Autodesk Fusion 360 part; units mm, degrees
sketch "Boceto1" plane through (0, 0, 0) normal (0, 1, 0) x (1, 0, 0)
  line L0 (3.025, -2.525) -> (16.025, -2.525)
  line L1 (3.025, -16.525) -> (16.025, -16.525)
  line L2 (2.525, -3.025) -> (2.525, -16.025)
  line L3 (16.525, -3.025) -> (16.525, -16.025)
  arc A0 (3.025, -2.525) -> (2.525, -3.025) centre (3.025, -3.025) ccw
  arc A1 (16.525, -3.025) -> (16.025, -2.525) centre (16.025, -3.025) ccw
  arc A2 (2.525, -16.025) -> (3.025, -16.525) centre (3.025, -16.025) ccw
  arc A3 (16.025, -16.525) -> (16.525, -16.025) centre (16.025, -16.025) ccw
  line L4 (22.075, -2.525) -> (35.075, -2.525)
  line L5 (22.075, -16.525) -> (35.075, -16.525)
  line L6 (21.575, -3.025) -> (21.575, -16.025)
  line L7 (35.575, -3.025) -> (35.575, -16.025)
  arc A4 (22.075, -2.525) -> (21.575, -3.025) centre (22.075, -3.025) ccw
  arc A5 (35.575, -3.025) -> (35.075, -2.525) centre (35.075, -3.025) ccw
  arc A6 (21.575, -16.025) -> (22.075, -16.525) centre (22.075, -16.025) ccw
  arc A7 (35.075, -16.525) -> (35.575, -16.025) centre (35.075, -16.025) ccw
  line L8 (3.025, -21.575) -> (16.025, -21.575)
  line L9 (3.025, -35.575) -> (16.025, -35.575)
  line L10 (2.525, -22.075) -> (2.525, -35.075)
  line L11 (16.525, -22.075) -> (16.525, -35.075)
  arc A8 (3.025, -21.575) -> (2.525, -22.075) centre (3.025, -22.075) ccw
  arc A9 (16.525, -22.075) -> (16.025, -21.575) centre (16.025, -22.075) ccw
  arc A10 (2.525, -35.075) -> (3.025, -35.575) centre (3.025, -35.075) ccw
  arc A11 (16.025, -35.575) -> (16.525, -35.075) centre (16.025, -35.075) ccw
  line L12 (22.075, -21.575) -> (35.075, -21.575)
  line L13 (22.075, -35.575) -> (35.075, -35.575)
  line L14 (21.575, -22.075) -> (21.575, -35.075)
  line L15 (35.575, -22.075) -> (35.575, -35.075)
  arc A12 (22.075, -21.575) -> (21.575, -22.075) centre (22.075, -22.075) ccw
  arc A13 (35.575, -22.075) -> (35.075, -21.575) centre (35.075, -22.075) ccw
  arc A14 (21.575, -35.075) -> (22.075, -35.575) centre (22.075, -35.075) ccw
  arc A15 (35.075, -35.575) -> (35.575, -35.075) centre (35.075, -35.075) ccw
  line L16 (-14.46, 33.91) -> (53.34, 33.91)
  line L17 (53.34, 33.91) -> (53.34, -52.19)
  line L18 (53.34, -52.19) -> (-14.46, -52.19)
  line L19 (-14.46, -52.19) -> (-14.46, 33.91)
  line L20 (10.09, 33.91) -> (28.59, 33.91)
  line L21 (28.59, 33.91) -> (28.59, 2.91)
  line L22 (28.59, 2.91) -> (10.09, 2.91)
  line L23 (10.09, 2.91) -> (10.09, 33.91)
  circle A16 centre (-9.46, 28.91) radius 1.7
  circle A17 centre (48.34, 28.91) radius 1.7
  circle A18 centre (-9.46, -47.19) radius 1.7
  circle A19 centre (48.34, -47.19) radius 1.7
  dimension "d1" = 86.1
  dimension "d2" = 67.8
  dimension "d3" = 16.615
  dimension "d4" = 16.985
  dimension "d5" = 17.765
  dimension "d6" = 18.5
  dimension "d7" = 31
  dimension "d8" = 24.55
  dimension "d9" = 3.4
  dimension "d10" = 3.4
  dimension "d11" = 3.4
  dimension "d12" = 3.4
  dimension "d13" = 5
  dimension "d14" = 5
  dimension "d15" = 5
  dimension "d16" = 5
  dimension "d17" = 5
  dimension "d18" = 5
  dimension "d19" = 5
  dimension "d20" = 5
extrude "Extruir1" add sketch "Boceto1" along normal blind 1.5 contours L16 L17 L18 L19 L21 L22 L23
fillet "Empalme1" radius 5 4 edges at (-14.46, 0.75, 52.19) (53.34, 0.75, 52.19) (-14.46, 0.75, -33.91) (53.34, 0.75, -33.91)
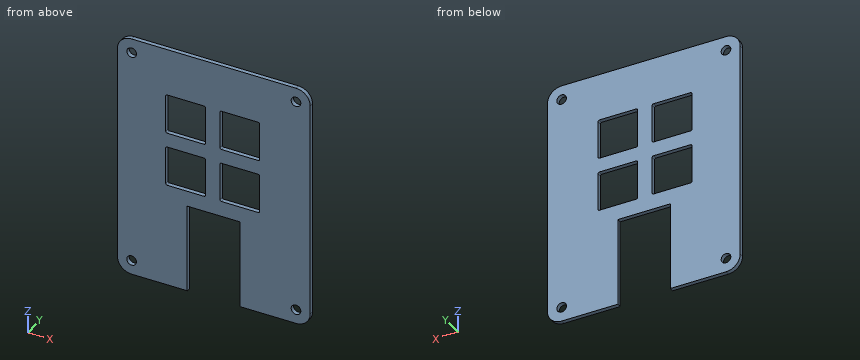
Geometry: final body of the model. Coordinates: model frame, mm. Round coordinates to 2 decimals unless told otherwise and drop trailing zeros. Loops run counter-clockwise (first coordinate to the right, second up) from the corner with the lowest first, then second, coordinate; pieces in that order, holes last.
Item 1: Section D-D, the plane y = 0.5. State how many separate pieces and enclosed holes the cut face has, plus the area to 3 significant figures.
Checked values:
separate pieces: 1
enclosed holes: 8
area: 4,420 mm2
Item 2: Contact query for a flat-ended pin moving along its axis: P1, Ø2, axis at x = 43, z = 15.5, coming from the -Y side. Output: stop coordinate, or through.
Checked values:
P1: stops at y = 0
Item 3: Section C-C, the plane z = 4.5. Output: boundary loops of the cut face in (x, y) (3 decimals).
Checked values:
outline: (-14.46, 0) - (2.525, 0) - (2.525, 1.5) - (-14.46, 1.5) - close; (16.525, 0) - (21.575, 0) - (21.575, 1.5) - (16.525, 1.5) - close; (35.575, 0) - (53.34, 0) - (53.34, 1.5) - (35.575, 1.5) - close
Item 4: Section B-B, the plane x = 8. Output: boundary loops of the cut face in (y, z) (3 decimals).
Checked values:
outline: (0, -33.91) - (1.5, -33.91) - (1.5, 2.525) - (0, 2.525) - close; (0, 16.525) - (1.5, 16.525) - (1.5, 21.575) - (0, 21.575) - close; (0, 35.575) - (1.5, 35.575) - (1.5, 52.19) - (0, 52.19) - close
Item 5: Line query: L1, parallel to Z at x = -9.46, y = 0.9; L2, parallel to Z at x = 3, y = 0.6; L3, parallel to X at y = 0.85, z = 47.19. Output: solid intervals per line, ascending.
Checked values:
L1: z = -33.91 to -30.61, -27.21 to 45.49, 48.89 to 52.19
L2: z = -33.91 to 2.53, 16.52 to 21.58, 35.57 to 52.19
L3: x = -14.46 to -11.16, -7.76 to 46.64, 50.04 to 53.34
Item 6: Section A-A, the plane z = -18.5. Output: boundary loops of the cut face in (x, y), plus the area to 4 significant figures.
Checked values:
outline: (-14.46, 0) - (10.09, 0) - (10.09, 1.5) - (-14.46, 1.5) - close; (28.59, 0) - (53.34, 0) - (53.34, 1.5) - (28.59, 1.5) - close
area: 73.95 mm2
